The model under review builds one solid part; all positions refer to its coordinate system, in mm. Face numbers are marked on the shaded views. A direction names the side the tool comes from. Give positions to 0.01 mm unless a question says otherwise; leave off trailing zeros. Loops run counter-clockwise (first coordinate to the right, second up) from the corner with the lowest first, then second, coordinate; pieces in that order, holes last. Notation, with made-up numbers: M -12.75,-13 L 21.25,-13 A24 ccw 21.25,19 Z; hole C -6.75,-8.75 d1. An arc over 180 degrees is marked long. Return JSON: item names as keys, results as strings. Group by question number.
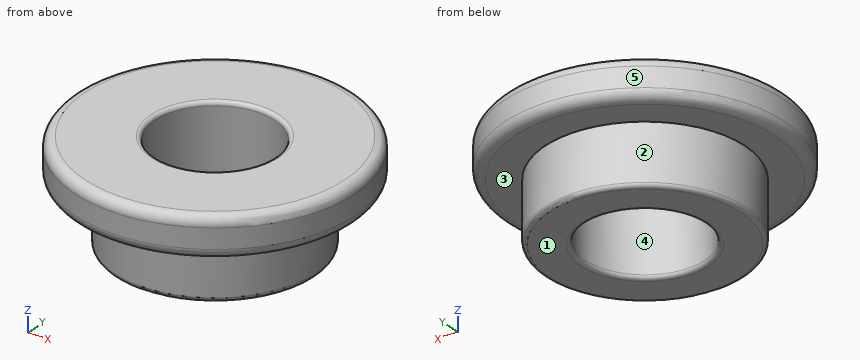
```python
from build123d import *

# Parameters (mm, degrees)
SKETCH_2_R                = 7
EXTRUDE_1_DEPTH           = 2
SKETCH_3_R                = 5
EXTRUDE_2_DEPTH           = 5
HOLE_WIZARD_6_0_6_1_D     = 6
HOLE_WIZARD_6_0_6_1_DEPTH = 30.32
HOLE_WIZARD_6_0_6_1_TIP   = 1.802581857
FILLET_1_R                = 0.5
FILLET_2_R                = 0.2


with BuildPart() as part:
    # 草图2 → 凸台-拉伸1 (new body)
    with BuildSketch(Plane.XY):
        Circle(SKETCH_2_R)
    extrude(amount=EXTRUDE_1_DEPTH)

    # 草图3 → 凸台-拉伸2 (add)
    with BuildSketch(Plane.XY.offset(2)):
        Circle(SKETCH_3_R)
    extrude(amount=-EXTRUDE_2_DEPTH)

    # Ø6.0 (6) 直径孔1
    with Locations(Plane.XY.offset(2)):
        with Locations((0, 0)):
            Hole(HOLE_WIZARD_6_0_6_1_D / 2, depth=HOLE_WIZARD_6_0_6_1_DEPTH)
            with Locations((0, 0, -(HOLE_WIZARD_6_0_6_1_DEPTH + HOLE_WIZARD_6_0_6_1_TIP / 2))):  # 118° drill point
                Cone(0, HOLE_WIZARD_6_0_6_1_D / 2, HOLE_WIZARD_6_0_6_1_TIP, mode=Mode.SUBTRACT)

    # 圆角1
    fillet_1_edges = [part.edges().sort_by_distance(p)[0] for p in [
        (-7, 0, 0),
        (-7, 0, 2),
    ]]
    fillet(fillet_1_edges, radius=FILLET_1_R)

    # 圆角2
    fillet_2_edges = [part.edges().sort_by_distance(p)[0] for p in [
        (3, 0, -3),
        (3, 0, 2),
        (-5, 0, -3),
    ]]
    fillet(fillet_2_edges, radius=FILLET_2_R)


solid = part.part
```
(1) For the marked faces 1 and 2, list the 3-axis set-ups (+Z, -Z, +X, -X, +Y, -Y) from which the entire face can be reached by the end or side of a thin tool; tool diameter is ignored.
(2) Mouldability with a two-part tool opening along X and no side actions: class the marked faces 3, 4 and 5 as released by +X, released by -X, zero draft, split by the parting line, or undercut.
(3) For pin 1 (2 mm diameter, centred on y = -5.5, z = -2, fed in from -X); pin 2 (2 mm diameter, centred on y = -5, z = -2.5, fed in from -X); pin 3 (5.5 mm diameter, centred on x = 0, y = 0, fed in from +Z); pin 4 (1 mm diameter, centred on y = 1.5, z = 0, fed in from -X), all flat-tipped, find the tip position at first contact; note any pin that passes through.
(4) Add section C-C (z = -1.05). Write out the cut boundary in (x, y), and give its area (3 significant figures).
(5) For probe 1 along Y at (x, z) = (0, -1.4); probe 2 along Y at (x, z) = (0, 0.45); probe 3 along X at (y, z) = (2, 0.6), list the stretches that pass through material, from the lowest coordinate up.
(6) Add section A-A (y = 0). Write out the cut boundary in (x, z).
Verdict:
{
 "1": {"face 1": "-Z, +X, -X, +Y, -Y", "face 2": "-Z"},
 "2": {"face 3": "zero draft", "face 4": "undercut", "face 5": "split by the parting line"},
 "3": {"pin 1": "stops at x = -2.18", "pin 2": "stops at x = -3", "pin 3": "passes through", "pin 4": "stops at x = -6.89"},
 "4": {"outline": "C 0,0 d10; hole C 0,0 d6", "area": "50.3 mm²"},
 "5": {"probe 1": "y = -5 to -3, 3 to 5", "probe 2": "y = -7 to -3, 3 to 7", "probe 3": "x = -6.71 to -2.24, 2.24 to 6.71"},
 "6": {"outline": "M -7,0.5 A0.5 ccw -6.5,0 L -5,0 L -5,-2.8 A0.2 ccw -4.8,-3 L -3.2,-3 A0.2 ccw -3,-2.8 L -3,1.8 A0.2 ccw -3.2,2 L -6.5,2 A0.5 ccw -7,1.5 Z; M 3,-2.8 A0.2 ccw 3.2,-3 L 4.8,-3 A0.2 ccw 5,-2.8 L 5,0 L 6.5,0 A0.5 ccw 7,0.5 L 7,1.5 A0.5 ccw 6.5,2 L 3.2,2 A0.2 ccw 3,1.8 Z"}
}
